Job drawing, mm, ordinate dimensions from the low corner. One solid piece. Give positions to 0.01 mm unless a question says otherwise; leave off trailing zeros. Order: outer loops, then holes, each group sorted by start corner. A loop starts at its lowest first (then second) coordinate and runs counter-clockwise, first axis right, second up. Notation, with made-up numbers: (40.25, 77.5) - (62.25, 77.5) arc R17 ccw to (62.25, 87.5) - close; hole circle Ø8 at (56.25, -12). An arc over 180 degrees is marked (long way). Write each question's results on one line, items separated by ' | '. Start each with the question number.
1) Cut at B-B on y = 0.65. State how many separate pieces and enclosed holes the cut face has, plus the area to 3 significant figures.
2) Drop flat-ended pins along their axis: pin 1 Ø1 at (y, z) = (1.5, 92.5) entering from -X; pin 2 Ø1.5 at (y, z) = (2, 12) entering from +X (1 decimal). Give the stop position or say it passes through.
3) Cut at C-C on x = 30. List the corners of the cut face in (y, z) (1 decimal).
4) Cut at A-A on z = 76.5. List the corners of the cut face in (x, y) (1 decimal).
5) Drill centre lines: line 1 along X through (y, z) = (0.4, 74) (1 decimal); line 2 along X through (y, z) = (2.8, 77) (1 decimal); line 3 along Z through (x, y) = (52, 1.4). Where is each one in solid material? Low to high. Write a range as from..to.
6) Cut at D-D on x = 57. List the corners of the cut face in (y, z) (1 decimal).
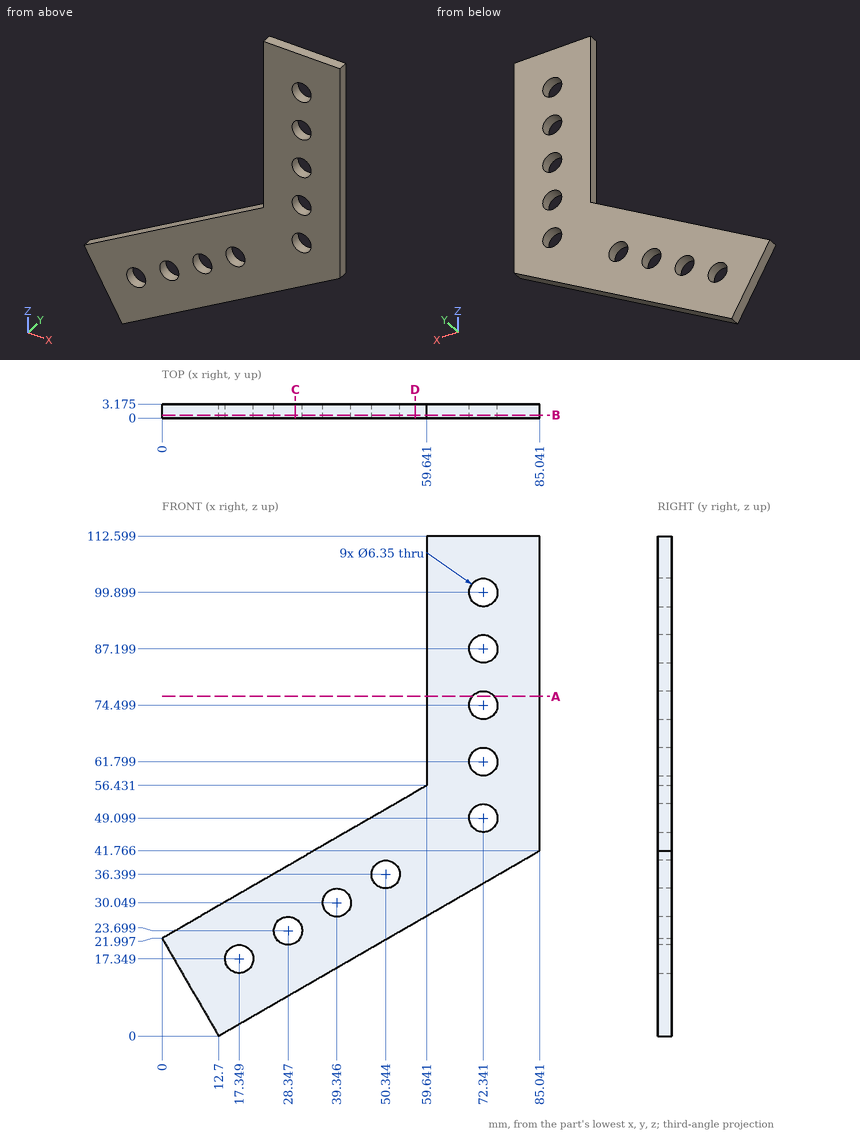
Results:
1) separate pieces: 1 | enclosed holes: 9 | area: 3,260 mm^2
2) pin 1: x = 59.64 | pin 2: x = 34.8
3) outline: (0, 10) - (3.2, 10) - (3.2, 21) - (0, 21) - close; (0, 26.4) - (3.2, 26.4) - (3.2, 39.3) - (0, 39.3) - close
4) outline: (59.6, 0) - (69.9, 0) - (69.9, 3.2) - (59.6, 3.2) - close; (74.8, 0) - (85, 0) - (85, 3.2) - (74.8, 3.2) - close
5) line 1: 59.6..69.2, 75.5..85 | line 2: 59.6..70.4, 74.3..85 | line 3: 22.69..33.69, 39.11..52.02
6) outline: (0, 25.6) - (3.2, 25.6) - (3.2, 54.9) - (0, 54.9) - close
